Check sheet for the modelled part. Datum: model origin and axes. Units: mm. Face numbers are marked on the shaded views. A direction names the side the tool comes from. Give positions to 0.01 mm unless a question says otherwise; leave off trailing zeros. Write each loop counter-clockwise with the first axis right and the second up, starting at its lowest first coordinate (ties: lowest second). Pieces come first, ordered by that corner, then holes.
from build123d import *

# Parameters (mm, degrees)
F0_R      = 11
F1_DEPTH  = 5
F2_R      = 2
F3_R      = 8
F3_R_2    = 6
F4_DEPTH  = 20
F4_FACE_R = 6
F5_DEPTH  = 35
F6_SIZE2  = 1
F6_SIZE   = 1
F7_W      = 1.5
F7_H      = 3
F8_DEPTH  = 12.5


with BuildPart() as f1:
    # F0 (on Front) → F1 (new body)
    with BuildSketch(Plane.XZ):
        Circle(F0_R)
    extrude(amount=F1_DEPTH)

    # F2
    f2_edges = [f1.edges().sort_by_distance(p)[0] for p in [
        (-11, -5, 0),
    ]]
    fillet(f2_edges, radius=F2_R)

    # F3 (on Front) → F4 (join)
    with BuildSketch(Plane.XZ):
        Circle(F3_R)
        Circle(F3_R_2, mode=Mode.SUBTRACT)
    extrude(amount=-F4_DEPTH)

    # F4_face (on face) → F5 (join)
    with BuildSketch(Plane(origin=(0, 0, 0), x_dir=(1, 0, 0), z_dir=(0, 1, 0))):
        Circle(F4_FACE_R)
    extrude(amount=F5_DEPTH)

    # F6
    f6_edges = [f1.edges().sort_by_distance(p)[0] for p in [
        (-6, 35, 0),
        (-8, 20, 0),
    ]]
    chamfer(f6_edges, length=F6_SIZE, length2=F6_SIZE2)

    # F7 (on Right) → F8 (cut, symmetric)
    with BuildSketch(Plane.YZ):
        with Locations((-4.25, 0)):
            Rectangle(F7_W, F7_H)
    extrude(amount=F8_DEPTH, both=True, mode=Mode.SUBTRACT)


solid = f1.part
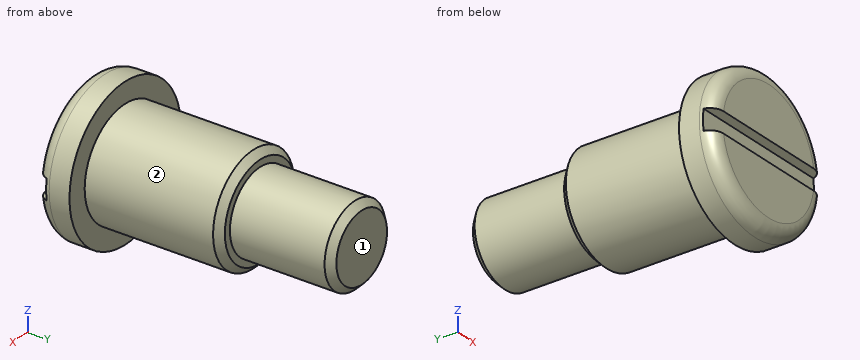
1) Access from +Z, -Z, +X, -X, +Y, -Y to the whole of each face (thin tool, end or side, straight path). Record for the marked faces 1 and 2.
2) Sectioned sample at A-A on z = 0. Record the boundary of the cut face in (x, y).
3) Sectioned sample at D-D on y = -1.5. Record the boundary of the cut face in (x, z).
4) Scan lines: L1, parallel to Y at x = 1.25, z = 0.25; L2, parallel to Z at x = 0, y = 30; L3, parallel to Y at x = 8.5, z = 0. Record each from-to range of solid material in increasing order.
5) Sectioned sample at B-B on x = 0. Record the boundary of the cut face in (y, z).
6) Sectioned sample at C-C on y = 29. Record the boundary of the cut face in (x, z).
7) Gauge pin test, flat ends, axial feed: pin 1 (1.2 mm diameter, centred on x = 3, y = -4.5, fed in from -Z); pin 2 (6 mm diameter, centred on x = -8.5, y = 12.5, fed in from +Z); pin 3 (11 mm diameter, centred on x = -4.5, z = 3.5, fed in from +Y); pin 4 (1.5 mm diameter, centred on y = 10, z = -5, fed in from -X). Record the tip position at first contact, or that the pin passes through.
Answers below:
1. face 1: +Z, -Z, +X, -X, +Y
1. face 2: +Y
2. outline: (-11, -3) arc R2 ccw to (-10.94, -3.5) - (10.94, -3.5) arc R2 ccw to (11, -3) - (11, 0) - (8, 0) - (8, 19) - (7, 20) - (6, 20) - (6, 34) - (5, 35) - (-5, 35) - (-6, 34) - (-6, 20) - (-7, 20) - (-8, 19) - (-8, 0) - (-11, 0) - close
3. outline: circle Ø22 at (0, 0)
4. L1: y = -3.5 to 35
4. L2: z = -6 to 6
4. L3: y = -3.5 to 0
5. outline: (-5, -9) arc R2 ccw to (-3, -11) - (0, -11) - (0, -8) - (19, -8) - (20, -7) - (20, -6) - (34, -6) - (35, -5) - (35, 5) - (34, 6) - (20, 6) - (20, 7) - (19, 8) - (0, 8) - (0, 11) - (-3, 11) arc R2 ccw to (-5, 9) - (-5, 1.5) - (-3.5, 1.5) - (-3.5, -1.5) - (-5, -1.5) - close
6. outline: circle Ø12 at (0, 0)
7. pin 1: stops at z = -10.4
7. pin 2: stops at z = 5.81
7. pin 3: stops at y = 35
7. pin 4: stops at x = -6.78
